For this review, take the finished solid that the model builds, in its own axes (mm). A direction names the side the tool comes from. Coordinates: 2 decimals unless noted, no trailing zeros. Loops run counter-clockwise (first coordinate to the right, second up) from the corner with the lowest first, then second, coordinate; pieces in that order, holes last. Notation, with made-up numbers: M 13.25,33 L 72.25,33 A21 cw 72.25,38 Z; hole C -37.75,45.5 d2. An arc over 180 degrees is marked long. Write each question's results on one line, items separated by ' | '. Start each with the question number.
Autodesk Inventor part; units mm, degrees
ref_plane "YZ Plane" through (0, 0, 0) normal (1, 0, 0) x (0, 1, 0)
ref_plane "XZ Plane" through (0, 0, 0) normal (0, 1, 0) x (-1, 0, 0)
ref_plane "XY Plane" through (0, 0, 0) normal (0, 0, 1) x (1, 0, 0)
sketch "Sketch1" plane through (0, 0, 0) normal (0, 1, 0) x (-1, 0, 0)
  line L0 (32.4676, 20.8715) -> (-27.5324, 20.8715)
  line L1 (-27.5324, 20.8715) -> (-27.5324, -46.1285)
  line L2 (-27.5324, -46.1285) -> (32.4676, -46.1285)
  line L3 (32.4676, -46.1285) -> (32.4676, 20.8715)
  point P0 (0, 0)
  dimension "d2" = 60
  dimension "d3" = 67
extrude "Extrusion1" add sketch "Sketch1" along normal blind 1
sketch "Sketch2" plane through (0, 1, 0) normal (0, 1, 0) x (1, 0, 0)
  line L0 (27.5324, 46.1285) -> (-32.4676, 46.1285)
  line L1 (-32.4676, 46.1285) -> (-32.4676, -20.8715)
  line L2 (27.5324, 46.1285) -> (-32.4676, 46.1285)
  line L3 (-32.4676, 46.1285) -> (-32.4676, 43.1285)
  line L4 (-32.4676, 43.1285) -> (27.5324, 43.1285)
  line L5 (27.5324, 43.1285) -> (27.5324, 46.1285)
  line L6 (27.5324, 46.1285) -> (24.5324, 46.1285)
  line L7 (24.5324, 46.1285) -> (24.5324, -13.8715)
  line L8 (24.5324, -13.8715) -> (27.5324, -13.8715)
  line L9 (27.5324, -13.8715) -> (27.5324, 46.1285)
  point P0 (0, 0)
  point P1 (24.5324, 43.1285)
  dimension "d8" = 3
  dimension "d9" = 3
extrude "Extrusion2" add sketch "Sketch2" along normal blind 20 contours L5 L4 L7 L0 | L7 L4 L1 L0
sketch "Sketch3" plane through (0, 21, 0) normal (0, 1, 0) x (1, 0, 0)
  line L0 (27.5324, 46.1285) -> (-32.4676, 46.1285)
  line L1 (-32.4676, 46.1285) -> (-32.4676, 43.1285)
  line L2 (-32.4676, 43.1285) -> (27.5324, 43.1285)
  line L3 (27.5324, 43.1285) -> (-32.4676, 43.1285)
  line L4 (-32.4676, 43.1285) -> (-32.4676, -20.8715)
  line L5 (-32.4676, -20.8715) -> (27.5324, -20.8715)
  line L6 (27.5324, 46.1285) -> (-32.4676, 46.1285)
  line L7 (27.5324, -20.8715) -> (27.5324, 46.1285)
  line L8 (-32.4676, 46.1285) -> (27.5324, 46.1285)
  line L9 (27.5324, 46.1285) -> (27.5324, 18.1285)
  line L10 (27.5324, 18.1285) -> (-32.4676, 18.1285)
  line L11 (-32.4676, 18.1285) -> (-32.4676, 46.1285)
  line L12 (-32.4676, 18.1285) -> (27.5324, 18.1285)
  line L13 (27.5324, 18.1285) -> (27.5324, 16.1285)
  line L14 (27.5324, 16.1285) -> (-32.4676, 16.1285)
  line L15 (-32.4676, 16.1285) -> (-32.4676, 18.1285)
  line L16 (27.5324, -20.8715) -> (27.5324, 43.1285)
  line L17 (27.5324, 43.1285) -> (27.5324, 46.1285)
  line L18 (-32.4676, 16.1285) -> (7.5324, 16.1285)
  line L19 (7.5324, 16.1285) -> (7.5324, -13.8715)
  line L20 (7.5324, -13.8715) -> (-32.4676, -13.8715)
  line L21 (-32.4676, -13.8715) -> (-32.4676, 16.1285)
  point P0 (0, 0)
  point P1 (-32.4676, 16.1285)
  point P2 (-32.4676, 18.1285)
  point P3 (-32.4676, -13.8715)
  dimension "d16" = 2
  dimension "d19" = 25
  dimension "d26" = 40
  dimension "d27" = 30
extrude "Extrusion3" add sketch "Sketch3" against normal blind 2 contours L7 L10 L4 L2 | L7 L14 L4 L10 | L14 L19 L20 L4
extrude "Extrusion5" add sketch "Sketch3" along normal blind 10 contours L7 L2 L1 L0 | L7 L14 L4 L10
sketch "Sketch5" plane through (27.5324, 0, -46.1285) normal (0, 0, -1) x (-1, 0, 0)
  circle A0 centre (10, 9.9562) radius 1
  circle A1 centre (50, 9.9562) radius 1
  line L0 (0, 0) -> (0, 31)
  point P0 (27.5324, 0)
  dimension "d20" = 2
  dimension "d21" = 2
  dimension "d22" = 40
  dimension "d23" = 10
extrude "Extrusion6" cut sketch "Sketch5" against normal blind 20
equation "\"d9\" = d8"
equation "\"d21\" = d20"
properties part number "electric_base"
Q1. Take a section at D-D, the plane y = 12.5. Give the boundary of the cut face in (x, z), then the cut area to 3 significant figures.
Q2. For faces 1 (the face through (-12, 20, 13.872)), 2 (the face through (-3, 26, -43.128)), 3 (the face through (7.532, 20, -1)), 4 (the face through (-2, 1, -11)), list the 3-axis set-ups (+Z, -Z, +X, -X, +Y, -Y) from which the entire face can be reached by the end or side of a thin tool; tool diameter is ignored.
Q3. The part is to be moulded in two halves that separate along X. For faces 5 (the face through (17.75, 8.98, -44.65)), 6 (the face through (27.532, 20, -27)), 7 (the face through (-13, 21, -1)), say which applies: pulls with the +X half, pulls with the -X half, needs draft (parallel to the pull), parting line crosses it, or undercut.
Q4. Take a section at B-B, the plane z = -37. Give the boundary of the cut face in (x, y).
Q5. Take a section at A-A, the plane y = 24. Give the boundary of the cut face in (x, z), then the cut area to 3 significant figures.
Q6. To check wall thickness, follow line 1 along Y through (x, z) = (-3.5, -32); line 2 along Z through (x, y) = (-3, 24); line 3 along Y through (x, z) = (14, -17.5). State the ranges of each line that lie inside material, in increasing order.
Q7. Take a section at C-C, the plane x = -3.5. Give the boundary of the cut face in (y, z).
Q8. Insertion check: P1, Ø2, axis at x = -13.5, y = 19.5, coming from the +Z side; P2, Ø2.5, axis at x = -22.47, y = 9.96, coming from the +Z side; P3, Ø7.5, axis at x = -2.5, z = -31.5, coming from the +Y side. Each pin has a flat end and moves straight along its axis. Give the tip position at first contact, or say it passes through.
Results:
1) outline: M -32.47,-46.13 L 27.53,-46.13 L 27.53,-43.13 L -32.47,-43.13 Z | area: 180 mm^2
2) face 1: +Z, +X, -X, +Y | face 2: +X, -X, +Y | face 3: +Z, +X, +Y | face 4: +Z, +X, -X
3) face 5: undercut | face 6: pulls with the +X half | face 7: needs draft
4) outline: M -32.47,0 L 27.53,0 L 27.53,1 L -32.47,1 Z; M -32.47,19 L 27.53,19 L 27.53,21 L -32.47,21 Z
5) outline: M -32.47,-46.13 L 27.53,-46.13 L 27.53,-43.13 L -32.47,-43.13 Z; M -32.47,-18.13 L 27.53,-18.13 L 27.53,-16.13 L -32.47,-16.13 Z | area: 300 mm^2
6) line 1: 0 to 1, 19 to 21 | line 2: -46.13 to -43.13, -18.13 to -16.13 | line 3: 0 to 1, 19 to 31
7) outline: M 0,-46.13 L 31,-46.13 L 31,-43.13 L 21,-43.13 L 21,-18.13 L 31,-18.13 L 31,-16.13 L 21,-16.13 L 21,13.87 L 19,13.87 L 19,-43.13 L 1,-43.13 L 1,20.87 L 0,20.87 Z
8) P1: z = 13.87 | P2: z = -43.13 | P3: y = 21
